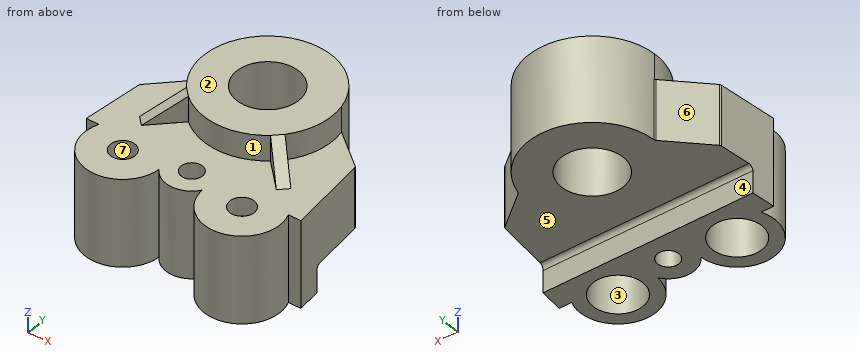
```python
from build123d import *

# Parameters (mm, degrees)
SALIENTE_EXTRUIR1_DEPTH      = 6.7
SALIENTE_EXTRUIR1_DEPTH_BACK = 5.5
CORTAR_EXTRUIR1_REACH        = 25.161
CROQUIS3_R                   = 3.35
CROQUIS3_R_2                 = 2.69
CROQUIS3_R_3                 = 1.15
CORTAR_EXTRUIR3_START        = -2.9
CORTAR_EXTRUIR3_DEPTH        = 2.9
CORTAR_EXTRUIR4_DEPTH        = 2.75
CROQUIS7_R                   = 4.1
CROQUIS7_R_2                 = 1.325
SALIENTE_EXTRUIR2_DEPTH      = 2.03
REDONDEO3_R                  = 0.5
REDONDEO4_R                  = 0.3
REDONDEO5_START              = -2.75
REDONDEO5_DEPTH              = 6.55
REDONDEO6_R                  = 0.3
REDONDEO7_R                  = 0.3
SALIENTE_EXTRUIR3_START      = 2.75
SALIENTE_EXTRUIR3_DEPTH      = 2.75
CORTAR_EXTRUIR5_REACH        = 23.382
CORTAR_EXTRUIR6_REACH        = 23.382
CROQUIS11_W                  = 25.480274204
CROQUIS11_H                  = 24.941512188
CORTAR_EXTRUIR7_DEPTH        = 33


with BuildPart() as part:
    # Croquis2 → Saliente-Extruir1 (new, two sides: drawn at the far end of the back side and taken through both)
    with BuildSketch(Plane.XY.offset(-SALIENTE_EXTRUIR1_DEPTH_BACK)):
        with BuildLine():
            Line((11.575, -10.275), (10.225721275, -10.275))
            ThreePointArc((10.225721275, -10.275), (7.338229527, -15.823139458), (2.337147732, -12.066992374))
            ThreePointArc((2.337147732, -12.066992374), (0, -13.325), (-2.337147732, -12.066992374))
            ThreePointArc((-2.337147732, -12.066992374), (-7.338229527, -15.823139458), (-10.225721275, -10.275))
            Line((-10.225721275, -10.275), (-11.575, -10.275))
            Line((-11.575, -10.275), (-10.892429135, -3.780772023))
            Line((-10.892429135, -3.780772023), (-6.911230699, 0.228287594))
            ThreePointArc((-6.911230699, 0.228287594), (-0.680469648, 6.88143779), (6.732669496, 1.577462032))
            Line((6.732669496, 1.577462032), (10.655149523, -1.523207321))
            Line((10.655149523, -1.523207321), (11.575, -10.275))
        make_face()
    extrude(amount=SALIENTE_EXTRUIR1_DEPTH + SALIENTE_EXTRUIR1_DEPTH_BACK)

    # Croquis3 → Cortar-Extruir1 (cut, up to next)
    with BuildSketch(Plane.XY.offset(6.7), mode=Mode.PRIVATE) as cortar_extruir1_sk1:
        Circle(CROQUIS3_R)
    cortar_extruir1_tool1 = extrude(cortar_extruir1_sk1.sketch, amount=-CORTAR_EXTRUIR1_REACH, mode=Mode.PRIVATE) & part.part
    # Croquis3 → Cortar-Extruir1 (cut, up to next)
    with BuildSketch(Plane.XY.offset(6.7), mode=Mode.PRIVATE) as cortar_extruir1_sk2:
        with Locations((6.43, -11.825)):
            Circle(CROQUIS3_R_2)
    cortar_extruir1_tool2 = extrude(cortar_extruir1_sk2.sketch, amount=-CORTAR_EXTRUIR1_REACH, mode=Mode.PRIVATE) & part.part
    # Croquis3 → Cortar-Extruir1 (cut, up to next)
    with BuildSketch(Plane.XY.offset(6.7), mode=Mode.PRIVATE) as cortar_extruir1_sk3:
        with Locations((-6.43, -11.825)):
            Circle(CROQUIS3_R_2)
    cortar_extruir1_tool3 = extrude(cortar_extruir1_sk3.sketch, amount=-CORTAR_EXTRUIR1_REACH, mode=Mode.PRIVATE) & part.part
    # Croquis3 → Cortar-Extruir1 (cut, up to next)
    with BuildSketch(Plane.XY.offset(6.7), mode=Mode.PRIVATE) as cortar_extruir1_sk4:
        with Locations((0, -10.525)):
            Circle(CROQUIS3_R_3)
    cortar_extruir1_tool4 = extrude(cortar_extruir1_sk4.sketch, amount=-CORTAR_EXTRUIR1_REACH, mode=Mode.PRIVATE) & part.part
    add(cortar_extruir1_tool1.solids().sort_by_distance((0, 0, 6.7))[0], mode=Mode.SUBTRACT)
    add(cortar_extruir1_tool2.solids().sort_by_distance((6.43, -11.825, 6.7))[0], mode=Mode.SUBTRACT)
    add(cortar_extruir1_tool3.solids().sort_by_distance((-6.43, -11.825, 6.7))[0], mode=Mode.SUBTRACT)
    add(cortar_extruir1_tool4.solids().sort_by_distance((0, -10.525, 6.7))[0], mode=Mode.SUBTRACT)

    # Croquis4 → Cortar-Extruir3 (cut)
    with BuildSketch(Plane.XY.offset(6.7).offset(CORTAR_EXTRUIR3_START)):
        with BuildLine():
            Line((-11.3069842, -7.725), (11.3069842, -7.725))
            Line((11.3069842, -7.725), (10.655149523, -1.523207321))
            Line((10.655149523, -1.523207321), (6.732669496, 1.577462032))
            ThreePointArc((6.732669496, 1.577462032), (-0.680469648, 6.88143779), (-6.911230699, 0.228287594))
            Line((-6.911230699, 0.228287594), (-10.892429135, -3.780772023))
            Line((-10.892429135, -3.780772023), (-11.3069842, -7.725))
        make_face()
    extrude(amount=CORTAR_EXTRUIR3_DEPTH, mode=Mode.SUBTRACT)

    # Croquis6 → Cortar-Extruir4 (cut)
    with BuildSketch(Plane(origin=(0, 0, -5.5), x_dir=(-1, 0, 0), z_dir=(0, 0, -1))):
        with BuildLine():
            Line((-11.575, -10.275), (-11.3069842, -7.725))
            Line((-11.3069842, -7.725), (-10.655149523, -1.523207321))
            Line((-10.655149523, -1.523207321), (-6.732669496, 1.577462032))
            ThreePointArc((-6.732669496, 1.577462032), (-0.680469648, -6.88143779), (6.911230699, 0.228287594))
            Line((6.911230699, 0.228287594), (10.892429135, -3.780772023))
            Line((10.892429135, -3.780772023), (11.3069842, -7.725))
            Line((11.3069842, -7.725), (11.575, -10.275))
            Line((11.575, -10.275), (10.225721275, -10.275))
            ThreePointArc((10.225721275, -10.275), (7.338229527, -15.823139458), (2.337147732, -12.066992374))
            ThreePointArc((2.337147732, -12.066992374), (0, -13.325), (-2.337147732, -12.066992374))
            ThreePointArc((-2.337147732, -12.066992374), (-7.338229527, -15.823139458), (-10.225721275, -10.275))
            Line((-10.225721275, -10.275), (-11.575, -10.275))
        make_face()
    extrude(amount=-CORTAR_EXTRUIR4_DEPTH, mode=Mode.SUBTRACT)

    # Croquis7 → Saliente-Extruir2 (add)
    # profile 1 of 2: a face of its own
    with BuildSketch(Plane(origin=(0, 0, -2.75), x_dir=(-1, 0, 0), z_dir=(0, 0, -1))):
        with Locations((-6.43, -11.825)):
            Circle(CROQUIS7_R)
        with Locations((-6.43, -11.825)):
            Circle(CROQUIS7_R_2, mode=Mode.SUBTRACT)
    # profile 2 of 2: a face of its own
    with BuildSketch(Plane(origin=(0, 0, -2.75), x_dir=(-1, 0, 0), z_dir=(0, 0, -1))):
        with Locations((6.43, -11.825)):
            Circle(CROQUIS7_R)
        with Locations((6.43, -11.825)):
            Circle(CROQUIS7_R_2, mode=Mode.SUBTRACT)
    extrude(amount=-SALIENTE_EXTRUIR2_DEPTH)

    # Redondeo3
    redondeo3_edges = [part.edges().sort_by_distance(p)[0] for p in [
        (0, -7.725, 3.8),
    ]]
    fillet(redondeo3_edges, radius=REDONDEO3_R)

    # Redondeo4
    redondeo4_edges = [part.edges().sort_by_distance(p)[0] for p in [
        (10.655149523, -1.523207321, 0.525),
    ]]
    fillet(redondeo4_edges, radius=REDONDEO4_R)

    # Redondeo5: read off the stored shape, not the designer's step
    # Redondeo5 outline → Redondeo5 (add)
    with BuildSketch(Plane.XY.offset(REDONDEO5_START)):
        with BuildLine():
            ThreePointArc((6.813852263, 1.513288112), (6.747864412, 1.585904369), (6.708836606, 1.675928518))
            ThreePointArc((6.708836606, 1.675928518), (6.720933379, 1.626738922), (6.732669496, 1.577462032))
            Line((6.732669496, 1.577462032), (6.813852263, 1.513288112))
        make_face()
    extrude(amount=REDONDEO5_DEPTH)

    # Redondeo6
    redondeo6_edges = [part.edges().sort_by_distance(p)[0] for p in [
        (-10.892429135, -3.780772023, 0.525),
    ]]
    fillet(redondeo6_edges, radius=REDONDEO6_R)

    # Redondeo7
    # the kernel refuses this fillet: 0.3 mm, written as the material it adds along each edge
    with BuildSketch(Plane(origin=(-6.911230699, 0.228287594, -2.75), x_dir=(-0.7046368913074451, -0.7095680738368798, 0), z_dir=(0, 0, 1))) as redondeo7_piece_1:
        with BuildLine():
            CenterArc((0.116455714, -0.3), REDONDEO7_R, 90, 41.963687937)
            ThreePointArc((-0.084142134, -0.076929376), (-0.041912521, -0.038638099), (0, 0))
            Line((0, 0), (0.116455714, 0))
        make_face()
    extrude(amount=6.55)

    # Croquis8 → Saliente-Extruir3 (add)
    with BuildSketch(Plane(origin=(0, 0, -2.75), x_dir=(-1, 0, 0), z_dir=(0, 0, -1)).offset(SALIENTE_EXTRUIR3_START)):
        with BuildLine():
            Line((7.718070517, -7.718070517), (7.276128778, -8.160012255))
            Line((7.276128778, -8.160012255), (4.427688638, -5.311572114))
            ThreePointArc((4.427688638, -5.311572114), (4.889643392, -4.889643392), (5.311572114, -4.427688638))
            Line((5.311572114, -4.427688638), (8.160012255, -7.276128778))
            Line((8.160012255, -7.276128778), (7.718070517, -7.718070517))
        make_face()
        with BuildLine():
            Line((-7.718070517, -7.718070517), (-7.276128778, -8.160012255))
            Line((-7.276128778, -8.160012255), (-4.427688638, -5.311572114))
            ThreePointArc((-4.427688638, -5.311572114), (-4.889643392, -4.889643392), (-5.311572114, -4.427688638))
            Line((-5.311572114, -4.427688638), (-8.160012255, -7.276128778))
            Line((-8.160012255, -7.276128778), (-7.718070517, -7.718070517))
        make_face()
    extrude(amount=-SALIENTE_EXTRUIR3_DEPTH)

    # Croquis9 → Cortar-Extruir5 (cut, up to next)
    with BuildSketch(Plane(origin=(-0.441941738, 0.441941738, 0), x_dir=(0, 0, 1), z_dir=(-0.7071067811865471, 0.7071067811865479, 0)), mode=Mode.PRIVATE) as cortar_extruir5_sk1:
        Polygon((-5.5, -6.886697322), (-2.75, -10.915), (-5.5, -10.915), align=None)
    cortar_extruir5_tool1 = extrude(cortar_extruir5_sk1.sketch, amount=-CORTAR_EXTRUIR5_REACH, mode=Mode.PRIVATE) & part.part
    add(cortar_extruir5_tool1.solids().sort_by_distance((-7.210532, -6.326649, -4.583333))[0], mode=Mode.SUBTRACT)

    # Croquis10 → Cortar-Extruir6 (cut, up to next)
    with BuildSketch(Plane(origin=(0.441941738, 0.441941738, 0), x_dir=(0, 0, -1), z_dir=(0.7071067811865479, 0.7071067811865472, 0)), mode=Mode.PRIVATE) as cortar_extruir6_sk1:
        Polygon((2.75, -10.915), (5.5, -10.915), (5.5, -6.886697322), align=None)
    cortar_extruir6_tool1 = extrude(cortar_extruir6_sk1.sketch, amount=-CORTAR_EXTRUIR6_REACH, mode=Mode.PRIVATE) & part.part
    add(cortar_extruir6_tool1.solids().sort_by_distance((7.210532, -6.326649, -4.583333))[0], mode=Mode.SUBTRACT)


with BuildPart() as body_2:
    # Simetría5: mirrored copy
    add(part.part.mirror(Plane(origin=(0, 0, -15.5), x_dir=(1, 0, 0), z_dir=(0, 0, -1))))


with BuildPart() as part_1:
    add(part.part)

    # Croquis11 → Cortar-Extruir7 (cut)
    with BuildSketch(Plane(origin=(0, 0, -15.5), x_dir=(-1, 0, 0), z_dir=(0, 0, -1))):
        with Locations((-0.09507565, -4.82477955)):
            Rectangle(CROQUIS11_W, CROQUIS11_H)
    extrude(amount=-CORTAR_EXTRUIR7_DEPTH, mode=Mode.SUBTRACT)


solid = body_2.part
```
Check sheet for the modelled part. Datum: model origin and axes. Units: mm. Face numbers are marked on the shaded views. A direction names the side the tool comes from. Round coordinates to 2 decimals unless told otherwise and drop trailing zeros. Loops run counter-clockwise (first coordinate to the right, second up) from the corner with the lowest first, then second, coordinate; pieces in that order, holes last. Notation, with made-up numbers: (72.5, -9) -> (122.5, -9) arc R20 cw to (122.5, 22) -> close; hole circle Ø10 at (-7.5, 41.5). An arc over 180 degrees is marked (long way). Answer in a Markdown table with one row per item.
Q1. Set-up check for the marked faces 1, 2, 3 and 4: record each of +Z, -Z, +X, -X, +Y, -Y from which the full face is reachable in a straight line by a thin tool's end or side.
Data:
| item | result |
|---|---|
| face 1 | +Z, -Y |
| face 2 | +Z, +X, -X, +Y, -Y |
| face 3 | -Z |
| face 4 | -Z, +X, -X, +Y |
Q2. Thickness scan on L1, parallel to Y at x = 0, z = -29 (3 decimals); L2, parallel to X at y = -10.5, z = -36.75; L3, parallel to X at y = -11, z = -32.25. Record the ranges inside material, lowest first.
Data:
| item | result |
|---|---|
| L1 | y = -13.325 to -11.675, -9.375 to -3.35, 3.35 to 6.915 |
| L2 | x = -10.31 to -8.77, -4.09 to -1.15, 1.15 to 4.09, 8.77 to 10.31 |
| L3 | x = -10.45 to -8.99, -3.87 to -1.05, 1.05 to 3.87, 8.99 to 10.45 |
Q3. Sectioned sample at C-C on z = -36.75. Enter the section's corners in (x, y) (3 decimals), then the cut area to 3 significant figures.
Data:
| item | result |
|---|---|
| outline | (-11.575, -10.275) -> (-10.226, -10.275) arc R4.1 ccw (long way) to (-2.337, -12.067) arc R2.8 ccw to (2.337, -12.067) arc R4.1 ccw (long way) to (10.226, -10.275) -> (11.575, -10.275) -> (11.307, -7.725) -> (-11.307, -7.725) -> close; hole circle Ø5.38 at (-6.43, -11.825); hole circle Ø2.3 at (0, -10.525); hole circle Ø5.38 at (6.43, -11.825) |
| area | 99.1 mm^2 |
Q4. Sectioned sample at D-D on x = -6.43. Enter the section's corners in (y, z) (3 decimals).
Data:
| item | result |
|---|---|
| outline | (-15.925, -37.7) -> (-14.515, -37.7) -> (-14.515, -30.28) -> (-13.15, -30.28) -> (-13.15, -28.25) -> (-15.925, -28.25) -> close; (-10.5, -30.28) -> (-9.135, -30.28) -> (-9.135, -37.7) -> (-7.725, -37.7) -> (-7.725, -35.3) arc R0.5 cw to (-7.225, -34.8) -> (2.544, -34.8) -> (2.544, -25.5) -> (-2.544, -25.5) -> (-2.544, -28.25) -> (-5.546, -28.25) -> (-5.546, -26.58) -> (-7.314, -27.433) -> (-7.314, -28.25) -> (-10.5, -28.25) -> close |
Q5. Go/stop test with flat-tipped pins: P1, Ø4, axis at x = -8, z = -35, coming from the +Y side; P2, Ø4.5, axis at x = 7.5, y = -11.5, coming from the -Z side; P3, Ø1.5, axis at x = 10.5, z = -32, coming from the -Y side; P4, Ø1.5, axis at x = 2.5, z = -28.5, coming from the +Y side. Record where each tip stops, or that it passes through.
Data:
| item | result |
|---|---|
| P1 | stops at y = 3.42 |
| P2 | stops at z = -37.7 |
| P3 | stops at y = -14.23 |
| P4 | stops at y = 6.69 |
Q6. Sectioned sample at B-B on y = 0.75. Enter the section's corners in (x, z).
Data:
| item | result |
|---|---|
| outline | (-6.87, -34.8) -> (-3.26, -34.8) -> (-3.26, -25.5) -> (-6.87, -25.5) -> close; (3.26, -34.8) -> (7.78, -34.8) -> (7.78, -28.25) -> (6.87, -28.25) -> (6.87, -25.5) -> (3.26, -25.5) -> close |
Q7. Release check for a two-part mould opening along Y. For the marked faces 5, 6 and 7 record: released by +Y, released by -Y, zero draft, split by the parting line, or undercut.
Data:
| item | result |
|---|---|
| face 5 | zero draft |
| face 6 | released by +Y |
| face 7 | undercut |
Q8. Sectioned sample at A-A on x = 0. Enter the section's corners in (y, z) (3 decimals).
Data:
| item | result |
|---|---|
| outline | (-13.325, -37.7) -> (-11.675, -37.7) -> (-11.675, -28.25) -> (-13.325, -28.25) -> close; (-9.375, -37.7) -> (-7.725, -37.7) -> (-7.725, -35.3) arc R0.5 cw to (-7.225, -34.8) -> (-3.35, -34.8) -> (-3.35, -25.5) -> (-6.915, -25.5) -> (-6.915, -28.25) -> (-9.375, -28.25) -> close; (3.35, -34.8) -> (6.915, -34.8) -> (6.915, -25.5) -> (3.35, -25.5) -> close |
